Verification items for the finished model (mm, model axes). A direction names the side the tool comes from. Round coordinates to 2 decimals unless told otherwise and drop trailing zeros. Write each loop counter-clockwise with the first axis right and the second up, starting at its lowest first coordinate (ties: lowest second). Pieces come first, ordered by that corner, then holes. Notation, with made-up numbers: (-14, 2) - (24, 2) arc R22 ccw to (24, 26) - close; hole circle Ø7 at (15, -8.75). An arc over 180 degrees is marked (long way). Answer as a JSON object with one key per item and string values.
```python
from build123d import *

# Parameters (mm, degrees)
SKETCH1_W           = 22
SKETCH1_H           = 13
BOSS_EXTRUDE1_DEPTH = 3


with BuildPart() as part:
    # Sketch1 → Boss-Extrude1 (new body)
    with BuildSketch(Plane.XY):
        Polygon((0, 29.9), (12.6, 29.9), (12.6, 32.9), (28.4, 32.9), (28.4, 29.9), (40.6, 29.9), (40.6, 32.9), (56.4, 32.9), (56.4, 29.9), (68.6, 29.9), (68.6, 32.9), (84.4, 32.9), (84.4, 29.9), (97, 29.9), (97, 22.95), (93.9, 22.95), (93.9, 6.95), (97, 6.95), (97, 0), (84.4, 0), (84.4, -3.1), (68.6, -3.1), (68.6, 0), (56.4, 0), (56.4, -3.1), (40.6, -3.1), (40.6, 0), (28.4, 0), (28.4, -3.1), (12.6, -3.1), (12.6, 0), (0, 0), (0, 6.95), (3.1, 6.95), (3.1, 22.95), (0, 22.95), align=None)
        with Locations((72.9, 20.4)):
            Rectangle(SKETCH1_W, SKETCH1_H, mode=Mode.SUBTRACT)
    extrude(amount=BOSS_EXTRUDE1_DEPTH)


solid = part.part
```
Q1. Section check C-C, the plane y = -1. Record the cut outline in (x, z), then the cut area to 3 significant figures.
Geometry check:
{"outline": "(12.6, 0) - (28.4, 0) - (28.4, 3) - (12.6, 3) - close; (40.6, 0) - (56.4, 0) - (56.4, 3) - (40.6, 3) - close; (68.6, 0) - (84.4, 0) - (84.4, 3) - (68.6, 3) - close", "area": "142 mm2"}
Q2. Section check D-D, the plane x = 88.5. Record the cut outline in (y, z), then the cut area to 3 significant figures.
Geometry check:
{"outline": "(0, 0) - (29.9, 0) - (29.9, 3) - (0, 3) - close", "area": "89.7 mm2"}
Q3. Material ranges on line 1 along Y through (x, z) = (63, 1.15); line 2 along Y through (x, z) = (83.5, 0.35); line 3 along X through (y, z) = (22, 1.3), recorded low to high. Write a range as [from, to].
Geometry check:
{"line 1": "y = [0, 13.9], [26.9, 29.9]", "line 2": "y = [-3.1, 13.9], [26.9, 32.9]", "line 3": "x = [3.1, 61.9], [83.9, 93.9]"}
Q4. Gauge pin test, flat ends, axial feed: P1, Ø0.9, axis at x = 67.5, z = 1, coming from the +Y side; P2, Ø0.9, axis at x = 62.5, z = 2, coming from the -Y side; P3, Ø0.9, axis at y = -2, z = 2, coming from the -X side. Record the tip position at first contact, or that the pin passes through.
Geometry check:
{"P1": "stops at y = 29.9", "P2": "stops at y = 0", "P3": "stops at x = 12.6"}
Q5. Section check B-B, the plane y = 25. Record the cut outline in (x, z), then the cut area to 3 significant figures.
Geometry check:
{"outline": "(0, 0) - (61.9, 0) - (61.9, 3) - (0, 3) - close; (83.9, 0) - (97, 0) - (97, 3) - (83.9, 3) - close", "area": "225 mm2"}
Q6. Set-up check for faces 1 (the flat face through (84.4, 31, 1)), 2 (the flat face through (40.6, -2, 1)), 3 (the flat face through (2, 6.95, 1)), 4 (the flat face through (40.6, 31, 1)), 5 (the flat face through (12.6, 31, 1)): record each of +Z, -Z, +X, -X, +Y, -Y from which the full face is reachable in a straight line by a thin tool's end or side.
Geometry check:
{"face 1": "+Z, -Z, +X, +Y", "face 2": "+Z, -Z, -Y", "face 3": "+Z, -Z, -X", "face 4": "+Z, -Z, +Y", "face 5": "+Z, -Z, -X, +Y"}
Q7. Section check A-A, the plane x = 73. Record the cut outline in (y, z).
Geometry check:
{"outline": "(-3.1, 0) - (13.9, 0) - (13.9, 3) - (-3.1, 3) - close; (26.9, 0) - (32.9, 0) - (32.9, 3) - (26.9, 3) - close"}
Q8. Release check for a two-part mould opening along Y. For faces 6 (the flat face through (93.9, 15, 1)), 7 (the flat face through (95, 6.95, 1)), 8 (the flat face through (91, 29.9, 1)), 9 (the flat face through (84.4, -2, 1)) record: released by +Y, released by -Y, zero draft, split by the parting line, or undercut.
Geometry check:
{"face 6": "undercut", "face 7": "undercut", "face 8": "released by +Y", "face 9": "zero draft"}
